Source: CAD feature listing. Evaluate the final solid. Frame: model axes, mm. A direction names the side the tool comes from. Coordinates: 2 decimals unless noted, no trailing zeros. Write each loop counter-clockwise with the first axis right and the second up, starting at its lowest first coordinate (ties: lowest second). Pieces come first, ordered by that corner, then holes. Notation, with made-up numbers: (-39, -36.75) -> (-16, -36.75) arc R33 cw to (-16, -3.75) -> close; hole circle Ø1 at (-17.75, 76.5). An arc over 180 degrees is marked (long way). One line per item, written item: value. Start each with the question number.
1. First-contact query: P1, Ø2.5, axis at x = -25, z = 79, coming from the -Y side; P2, Ø1.5, axis at x = 6.5, y = -1.5, coming from the +Z side; P3, Ø4, axis at y = -2.5, z = 56, coming from the +X side. Flat tips, straight axial feed; report the tip coordinate or a pass-through.
2. Section query A-A, the plane x = -25. Output: boundary loops of the cut face in (y, z).
3. Section query C-C, the plane x = -12. Output: boundary loops of the cut face in (y, z).
4. Access query for faces 4 (the flat face through (-20, -4, 57)), 5 (the flat face through (-15, -4, -27)). Directions: +Z, -Z, +X, -X, +Y, -Y. A direction counts if a zero-diameter tool reaches every point of the face in a straight line with its end or side. Return the directions, or none.
5. Mould query, pull axis Z, two halves, no side actions, for faces 1 (the flat face through (-7, -4, 27)), 2 (the cylindrical face through (9.2, -3.9, 17.7)), 3 (the flat face through (-32, 0, 29)). Classes: released by +Z, released by -Z, zero draft, split by the parting line, or undercut.
6. Section query D-D, the plane x = -45. Output: boundary loops of the cut face in (y, z).
7. Line query: line 1 (Z direction, x = 0, y = -6); line 2 (X direction, y = -5.25, z = -18.5); line 3 (Z direction, x = 13, y = -5.25). Output: solid intervals per line, ascending.
8. Section query B-B, the plane y = -5.25. Output: boundary loops of the cut face in (x, z).
from build123d import *

# Parameters (mm, degrees)
F0_R     = 2.25
F0_R_2   = 1.6
F1_DEPTH = 8


with BuildPart() as f1:
    # F0 (on Front) → F1 (new body)
    with BuildSketch(Plane.XZ):
        with BuildLine():
            ThreePointArc((9.298187, -14.351087), (-17.1, 0), (9.298187, 14.351087))
            ThreePointArc((9.298187, 14.351087), (15.5334, 16.943464), (13.5, 23.382686))
            ThreePointArc((13.5, 23.382686), (6.988114, 26.079997), (0, 27))
            Line((0, 27), (-15, 27))
            ThreePointArc((-15, 27), (-18.535534, 28.464466), (-20, 32))
            Line((-20, 32), (-20, 83))
            Line((-20, 83), (-50, 83))
            Line((-50, 83), (-50, -7))
            ThreePointArc((-50, -7), (-44.142136, -21.142136), (-30, -27))
            Line((-30, -27), (0, -27))
            ThreePointArc((0, -27), (6.988114, -26.079997), (13.5, -23.382686))
            ThreePointArc((13.5, -23.382686), (15.5334, -16.943464), (9.298187, -14.351087))
        make_face()
        with Locations((-11, -19.052559)):
            Circle(F0_R, mode=Mode.SUBTRACT)
        with Locations((11, -19.052559)):
            Circle(F0_R, mode=Mode.SUBTRACT)
        with Locations((-11, 19.052559)):
            Circle(F0_R, mode=Mode.SUBTRACT)
        with Locations((11, 19.052559)):
            Circle(F0_R, mode=Mode.SUBTRACT)
        with Locations((-45, 79)):
            Circle(F0_R_2, mode=Mode.SUBTRACT)
        with Locations((-25, 79)):
            Circle(F0_R_2, mode=Mode.SUBTRACT)
    extrude(amount=F1_DEPTH)


solid = f1.part
Computed values:
1. P1: passes through
1. P2: stops at z = 26.38
1. P3: stops at x = -20
2. outline: (-8, -27) -> (0, -27) -> (0, 77.4) -> (-8, 77.4) -> close; (-8, 80.6) -> (0, 80.6) -> (0, 83) -> (-8, 83) -> close
3. outline: (-8, -27) -> (0, -27) -> (0, -21.07) -> (-8, -21.07) -> close; (-8, -17.04) -> (0, -17.04) -> (0, -12.18) -> (-8, -12.18) -> close; (-8, 12.18) -> (0, 12.18) -> (0, 17.04) -> (-8, 17.04) -> close; (-8, 21.07) -> (0, 21.07) -> (0, 27) -> (-8, 27) -> close
4. face 4: +Z, +X, +Y, -Y
4. face 5: -Z, +X, -X, +Y, -Y
5. face 1: released by +Z
5. face 2: undercut
5. face 3: zero draft
6. outline: (-8, -20.23) -> (0, -20.23) -> (0, 77.4) -> (-8, 77.4) -> close; (-8, 80.6) -> (0, 80.6) -> (0, 83) -> (-8, 83) -> close
7. line 1: z = -27 to -17.1, 17.1 to 27
7. line 2: x = -46.36 to -13.18, -8.82 to 8.82, 13.18 to 15.97
7. line 3: z = -23.66 to -20.08, -18.02 to -14.47, 14.47 to 18.02, 20.08 to 23.66
8. outline: (-50, -7) arc R20 ccw to (-30, -27) -> (0, -27) arc R27 ccw to (13.5, -23.38) arc R5 ccw to (9.3, -14.35) arc R17.1 cw (long way) to (9.3, 14.35) arc R5 ccw to (13.5, 23.38) arc R27 ccw to (0, 27) -> (-15, 27) arc R5 cw to (-20, 32) -> (-20, 83) -> (-50, 83) -> close; hole circle Ø3.2 at (-45, 79); hole circle Ø3.2 at (-25, 79); hole circle Ø4.5 at (-11, -19.05); hole circle Ø4.5 at (-11, 19.05); hole circle Ø4.5 at (11, -19.05); hole circle Ø4.5 at (11, 19.05)
